from build123d import *

# Parameters (mm, degrees)
SKETCH_1_W          = 43
SKETCH_1_H          = 40
EXTRUDE_1_DEPTH     = 8
SKETCH_2_R          = 1.3
CUT_EXTRUDE_1_DEPTH = 8
CHAMFER_1_SIZE      = 0.2


with BuildPart() as part:
    # 草圖1 → 填料-伸長1 (new body)
    with BuildSketch(Plane(origin=(0, 0, 0), x_dir=(1, 0, 0), z_dir=(0, 1, 0))):
        Rectangle(SKETCH_1_W, SKETCH_1_H)
    extrude(amount=EXTRUDE_1_DEPTH)

    # 草圖2 → 除料-伸長1 (cut)
    with BuildSketch(Plane.ZY.offset(21.5)):
        with Locations((-12, 4)):
            Circle(SKETCH_2_R)
        with Locations((12, 4)):
            Circle(SKETCH_2_R)
    cut_extrude_1 = extrude(amount=-CUT_EXTRUDE_1_DEPTH, mode=Mode.SUBTRACT)

    # 鏡射1: 除料-伸長1 across plane
    add(cut_extrude_1.mirror(Plane(origin=(0, 0, 0), x_dir=(0, 0, 1), z_dir=(1, 0, 0))), mode=Mode.SUBTRACT)

    # 導角1
    chamfer_1_edges = [part.edges().sort_by_distance(p)[0] for p in [
        (-21.5, 4, -13.3),
        (-21.5, 4, 10.7),
        (21.5, 4, -13.3),
        (21.5, 4, 10.7),
    ]]
    chamfer(chamfer_1_edges, length=CHAMFER_1_SIZE)


solid = part.part
Geometry: final body of the model. Coordinates: model frame, mm. A direction names the side the tool comes from. Coordinates: 2 decimals unless noted, no trailing zeros. Loops run counter-clockwise (first coordinate to the right, second up) from the corner with the lowest first, then second, coordinate; pieces in that order, holes last. Notation, with made-up numbers: M 11,35 L 45,35 A8 cw 45,40 Z; hole C 25,67 d1. An arc over 180 degrees is marked long. One line per item, written item: value. Start each with the question number.
1) Draft query along Z for faces 4 (the flat face through (0, 4, 20)), 5 (the cylindrical face through (17.455, 2.847, -11.4)), 6 (the flat face through (0, 0, 0)). Return one class per face: released by +Z, released by -Z, zero draft, split by the parting line, or undercut.
2) Material intervals for L1, parallel to Y at x = 18, z = 12, sorted ascending. Write a range as from..to.
3) Cut plane C-C (z = 12). Return loops of the section in (x, y), then the cut area to 3 significant figures.
4) Reachability of faces 1 (the cylindrical face through (-17.455, 2.847, 12.6)), 2 (the flat face through (0, 4, -20)), 3 (the flat face through (13.5, 4, -12)) from +Z, -Z, +X, -X, +Y, -Y: full face, straight path, thin tool, end or side. Return the list, or none.
5) Cut plane B-B (x = -18). Return loops of the section in (y, z), then the cut area to 3 significant figures.
6) Cut plane A-A (y = 4). Return loops of the section in (x, z), then the cut area to 3 significant figures.
7) Pin query (flat end, axial travel): P1, Ø1.3, axis at y = 4.5, z = 12, coming from the +X side; P2, Ø0.8, axis at y = 4.5, z = 11.5, coming from the -X side. Return the tip coordinate at first contact, or that it passes through.
Evaluation:
1. face 4: released by +Z
1. face 5: undercut
1. face 6: zero draft
2. L1: 0..2.7, 5.3..8
3. outline: M -21.5,0 L 21.5,0 L 21.5,2.5 L 21.3,2.7 L 13.5,2.7 L 13.5,5.3 L 21.3,5.3 L 21.5,5.5 L 21.5,8 L -21.5,8 L -21.5,5.5 L -21.3,5.3 L -13.5,5.3 L -13.5,2.7 L -21.3,2.7 L -21.5,2.5 Z
3. area: 302 mm^2
4. face 1: -X
4. face 2: -Z, +X, -X, +Y, -Y
4. face 3: +X
5. outline: M 0,-20 L 8,-20 L 8,20 L 0,20 Z; hole C 4,-12 d2.6; hole C 4,12 d2.6
5. area: 309 mm^2
6. outline: M -21.5,-20 L 21.5,-20 L 21.5,-13.5 L 21.3,-13.3 L 13.5,-13.3 L 13.5,-10.7 L 21.3,-10.7 L 21.5,-10.5 L 21.5,10.5 L 21.3,10.7 L 13.5,10.7 L 13.5,13.3 L 21.3,13.3 L 21.5,13.5 L 21.5,20 L -21.5,20 L -21.5,13.5 L -21.3,13.3 L -13.5,13.3 L -13.5,10.7 L -21.3,10.7 L -21.5,10.5 L -21.5,-10.5 L -21.3,-10.7 L -13.5,-10.7 L -13.5,-13.3 L -21.3,-13.3 L -21.5,-13.5 Z
6. area: 1,640 mm^2
7. P1: x = 13.5
7. P2: x = -13.5
